from build123d import *

# Parameters (mm, degrees)
SKETCH_R  = 11
PAD_DEPTH = 7
FILLET_R  = 3


with BuildPart() as part:
    # Sketch → Pad (new body)
    with BuildSketch(Plane.XY):
        with BuildLine():
            ThreePointArc((24.736194, -2.705303), (32.908969, 18.999993), (10.025247, 22.774834))
            ThreePointArc((-10.025222, 22.774812), (1.7e-05, 19), (10.025247, 22.774834))
            ThreePointArc((-10.025222, 22.774812), (-32.908957, 19.000015), (-24.736208, -2.705298))
            ThreePointArc((-14.71096, -20.069529), (-16.454484, -9.499997), (-24.736208, -2.705298))
            ThreePointArc((-14.71096, -20.069529), (-4e-06, -38), (14.710962, -20.069538))
            ThreePointArc((24.736194, -2.705303), (16.454478, -9.500007), (14.710962, -20.069538))
        make_face()
        with Locations((-19.918584, 11.5)):
            Circle(SKETCH_R, mode=Mode.SUBTRACT)
        Circle(SKETCH_R, mode=Mode.SUBTRACT)
        with Locations((19.918584, 11.5)):
            Circle(SKETCH_R, mode=Mode.SUBTRACT)
        with Locations((0, -23)):
            Circle(SKETCH_R, mode=Mode.SUBTRACT)
    extrude(amount=PAD_DEPTH)

    # Fillet
    fillet_edges = [part.edges().sort_by_distance(p)[0] for p in [
        (32.908969, 18.999993, 0),
        (32.908969, 18.999993, 7),
    ]]
    fillet(fillet_edges, radius=FILLET_R)


solid = part.part
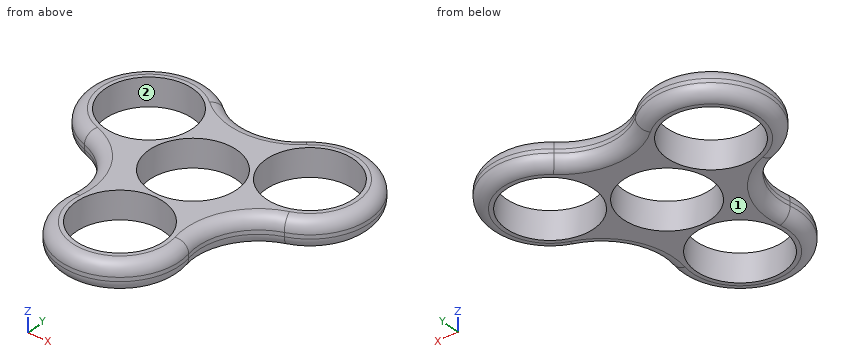
Model file for the job. Use its own axes, mm. Face numbers are marked on the shaded views. Give positions to 0.01 mm unless a question says otherwise; leave off trailing zeros. Loops run counter-clockwise (first coordinate to the right, second up) from the corner with the lowest first, then second, coordinate; pieces in that order, holes last.
1) Saw through at C-C (z = 5.25). Write the cut outline in (x, y), plus the area to 3 significant figures.
2) Flat gauge pins, fed straight in: pin 1 Ø13 at (x, y) = (-19.92, 11.5) entering from -Z; pin 2 Ø8 at (x, y) = (-16, -15) entering from -Z; pin 3 Ø3 at (y, z) = (15, 1.5) entering from +X; pin 4 Ø2 at (x, z) = (-17.5, 1.5) entering from -Y. Where does each tip first touch, or does it go through?
3) Pull direction Y, two halves, no side cores. Call the marked faces 1 and 2: +Y half, -Y half, draft (parallel to the pull), parting line (faces both ways), or undercut.
4) Saw through at A-A (z = 1.5). Write the cut outline in (x, y), plus the area to 3 significant figures.
5) Wall check: line 1 (Y direction, x = 4.5, z = 0.5); line 2 (X direction, y = 1.5, z = 4.75); line 3 (Y direction, x = 5, z = 1.75). Give the ranges that are in metal, low to high.
6) Saw through at B-B (x = 0). Count the separate pieces of the cut face and the enclosed holes in it, plus the area to 3 significant figures.
Answer block:
1. outline: (-24.65, -2.45) arc R15.47 cw to (-14.44, -20.12) arc R14.73 ccw (long way) to (14.44, -20.12) arc R15.47 cw to (24.65, -2.45) arc R14.73 ccw (long way) to (10.21, 22.57) arc R15.47 cw to (-10.21, 22.57) arc R14.73 ccw (long way) to start; hole circle Ø22 at (-19.92, 11.5); hole circle Ø22 at (0, -23); hole circle Ø22 at (0, 0); hole circle Ø22 at (19.92, 11.5)
1. area: 1,160 mm2
2. pin 1: passes through
2. pin 2: stops at z = 0.03
2. pin 3: stops at x = 34.69
2. pin 4: stops at y = -8.88
3. face 1: draft
3. face 2: undercut
4. outline: (-24.61, -2.32) arc R15.6 cw to (-14.32, -20.15) arc R14.6 ccw (long way) to (14.32, -20.15) arc R15.6 cw to (24.61, -2.32) arc R14.6 ccw (long way) to (10.29, 22.47) arc R15.6 cw to (-10.29, 22.47) arc R14.6 ccw (long way) to start; hole circle Ø22 at (-19.92, 11.5); hole circle Ø22 at (0, -23); hole circle Ø22 at (0, 0); hole circle Ø22 at (19.92, 11.5)
4. area: 1,130 mm2
5. line 1: y = -35.9 to -33.04, -12.96 to -10.04, 10.04 to 18.28
5. line 2: x = -30.97 to -24.5, -15.34 to -10.9, 10.9 to 15.34, 24.5 to 30.97
5. line 3: y = -36.85 to -32.8, -13.2 to -9.8, 9.8 to 19.56
6. separate pieces: 3
6. enclosed holes: 0
6. area: 83.3 mm2
